Check sheet for the modelled part. Datum: model origin and axes. Units: mm. A direction names the side the tool comes from. Round coordinates to 2 decimals unless told otherwise and drop trailing zeros. Order: outer loops, then holes, each group sorted by start corner. A loop starts at its lowest first (then second) coordinate and runs counter-clockwise, first axis right, second up.
```python
from build123d import *

# Parameters (mm, degrees)
BOSS_EXTRUDE1_DEPTH = 20
FILLET1_R           = 10
SKETCH2_R           = 4
SKETCH2_R_2         = 1.9
BOSS_EXTRUDE2_DEPTH = 5
SKETCH3_R           = 1.9
CUT_EXTRUDE1_DEPTH  = 52.478150705
SKETCH5_R           = 4
SKETCH5_R_2         = 1.9
BOSS_EXTRUDE3_DEPTH = 5
SKETCH6_R           = 1.9
CUT_EXTRUDE2_DEPTH  = 44.874821937
FILLET2_R           = 2


with BuildPart() as part:
    # Sketch1 → Boss-Extrude1 (new body)
    with BuildSketch(Plane(origin=(0, 0, 0), x_dir=(1, 0, 0), z_dir=(0, 1, 0))):
        Polygon((-20, 15), (20, 15), (20, -15), (15.05, -15), (15.05, 10), (-15.05, 10), (-15.05, -15), (-20, -15), align=None)
    extrude(amount=BOSS_EXTRUDE1_DEPTH)

    # Fillet1
    fillet1_edges = [part.edges().sort_by_distance(p)[0] for p in [
        (-20, 10, -15),
        (20, 10, -15),
        (15.05, 10, -10),
        (-15.05, 10, -10),
    ]]
    fillet(fillet1_edges, radius=FILLET1_R)

    # Sketch2 → Boss-Extrude2 (add)
    with BuildSketch(Plane(origin=(20, 0, 0), x_dir=(0, 0, -1), z_dir=(1, 0, 0))):
        with Locations(Location((-5, 10, 0), (0, 0, 180))):
            Circle(SKETCH2_R)
        with Locations((-5, 10)):
            Circle(SKETCH2_R_2, mode=Mode.SUBTRACT)
    boss_extrude2 = extrude(amount=BOSS_EXTRUDE2_DEPTH)

    # Mirror1: Boss-Extrude2 across plane
    add(boss_extrude2.mirror(Plane(origin=(0, 0, 0), x_dir=(0, 0, 1), z_dir=(1, 0, 0))))

    # Sketch3 → Cut-Extrude1 (cut, through all)
    with BuildSketch(Plane(origin=(20, 0, 0), x_dir=(0, 0, -1), z_dir=(1, 0, 0))):
        with Locations((-5, 10)):
            Circle(SKETCH3_R)
    extrude(amount=-CUT_EXTRUDE1_DEPTH, mode=Mode.SUBTRACT)

    # Sketch5 → Boss-Extrude3 (add)
    with BuildSketch(Plane(origin=(0, 0, -15), x_dir=(-1, 0, 0), z_dir=(0, 0, -1))):
        with Locations(Location((0, 10, 0), (0, 0, 180))):
            Circle(SKETCH5_R)
        with Locations((0, 10)):
            Circle(SKETCH5_R_2, mode=Mode.SUBTRACT)
    extrude(amount=BOSS_EXTRUDE3_DEPTH)

    # Sketch6 → Cut-Extrude2 (cut, through all)
    with BuildSketch(Plane(origin=(0, 0, -15), x_dir=(-1, 0, 0), z_dir=(0, 0, -1))):
        with Locations((0, 10)):
            Circle(SKETCH6_R)
    extrude(amount=-CUT_EXTRUDE2_DEPTH, mode=Mode.SUBTRACT)

    # Fillet2
    fillet2_edges = [part.edges().sort_by_distance(p)[0] for p in [
        (-15.05, 0, 7.5),
        (-17.525, 0, 15),
        (-20, 0, 5),
        (0, 0, -15),
        (15.05, 0, 7.5),
        (0, 0, -10),
        (17.071067812, 0, -12.071067812),
        (-17.071067812, 0, -12.071067812),
        (12.121067812, 0, -7.071067812),
        (-12.121067812, 0, -7.071067812),
        (20, 0, 5),
        (17.525, 0, 15),
    ]]
    fillet(fillet2_edges, radius=FILLET2_R)


solid = part.part
```
Item 1: Access from +Z, -Z, +X, -X, +Y, -Y to the whole of each face (thin tool, end or side, straight path). Record for faces 4 (the cylindrical face through (-0.07, 0.57, -10.6)), 5 (the flat face through (25, 11, 7)), 6 (the cylindrical face through (-22.465, 13.905, 4.133)), 7 (the flat face through (2, 11, -20)), 8 (the cylindrical face through (12.2, 11.13, -6.99)).
Answer:
face 4: +Z, -Y
face 5: +Z, -Z, +X, +Y, -Y
face 6: -X
face 7: -Z, +X, -X, +Y, -Y
face 8: +Z, +Y, -Y
Item 2: Go/stop test with flat-tipped pins: P1, Ø3.5, axis at x = 0, y = 10, coming from the +Z side; P2, Ø1, axis at x = -12.5, y = 5, coming from the +Z side; P3, Ø6, axis at x = 18, y = 11, coming from the -Z side; P4, Ø2, axis at y = 17.5, z = 2, coming from the +X side. Record where each tip stops, or that it passes through.
Answer:
P1: passes through
P2: stops at z = -6.07
P3: stops at z = -13.66
P4: stops at x = 20
Item 3: Sectioned sample at C-C (y = 3.5). Record the cut outline in (x, z).
Answer:
outline: (-20, -5) arc R10 ccw to (-10, -15) - (10, -15) arc R10 ccw to (20, -5) - (20, 15) - (15.05, 15) - (15.05, 0) arc R10 cw to (5.05, -10) - (-5.05, -10) arc R10 cw to (-15.05, 0) - (-15.05, 15) - (-20, 15) - close
Item 4: Sectioned sample at B-B (z = 5). Record the cut outline in (x, y).
Answer:
outline: (-25, 6) - (-20, 6) - (-20, 2) arc R2 ccw to (-18, 0) - (-17.05, 0) arc R2 ccw to (-15.05, 2) - (-15.05, 8.1) - (-25, 8.1) - close; (-25, 11.9) - (-15.05, 11.9) - (-15.05, 20) - (-20, 20) - (-20, 14) - (-25, 14) - close; (15.05, 2) arc R2 ccw to (17.05, 0) - (18, 0) arc R2 ccw to (20, 2) - (20, 6) - (25, 6) - (25, 8.1) - (15.05, 8.1) - close; (15.05, 11.9) - (25, 11.9) - (25, 14) - (20, 14) - (20, 20) - (15.05, 20) - close
Item 5: Release check for a two-part mould opening along X. For faces 1 (the cylindrical face through (-12.04, 11.13, -7.15)), 2 (the cylindrical face through (-17.6, 0.8, 14.6)), 3 (the cylindrical face through (-0.867, 13.905, -17.465)) record: released by +X, released by -X, zero draft, split by the parting line, or undercut.
Answer:
face 1: undercut
face 2: zero draft
face 3: split by the parting line
Item 6: Scan lines: line 1 along Y through (x, z) = (0, -17.85); line 2 along X through (y, z) = (7, 13); line 3 along X through (y, z) = (13, 4). Record each from-to range of solid material in increasing order.
Answer:
line 1: y = 6 to 8.1, 11.9 to 14
line 2: x = -20 to -15.05, 15.05 to 20
line 3: x = -25 to -15.05, 15.05 to 25
Item 7: Sectioned sample at A-A (x = 0). Record the cut outline in (y, z).
Answer:
outline: (0, -13) arc R2 ccw to (2, -15) - (6, -15) - (6, -20) - (8.1, -20) - (8.1, -10) - (2, -10) arc R2 ccw to (0, -12) - close; (11.9, -20) - (14, -20) - (14, -15) - (20, -15) - (20, -10) - (11.9, -10) - close
Item 8: Sectioned sample at D-D (y = 12.75). Record the cut outline in (x, z), and give its area (3 significant figures).
Answer:
outline: (-25, 2.1) - (-20, 2.1) - (-20, -5) arc R10 ccw to (-10, -15) - (-2.9, -15) - (-2.9, -20) - (2.9, -20) - (2.9, -15) - (10, -15) arc R10 ccw to (20, -5) - (20, 2.1) - (25, 2.1) - (25, 7.9) - (20, 7.9) - (20, 15) - (15.05, 15) - (15.05, 0) arc R10 cw to (5.05, -10) - (-5.05, -10) arc R10 cw to (-15.05, 0) - (-15.05, 15) - (-20, 15) - (-20, 7.9) - (-25, 7.9) - close
area: 535 mm2
